Source: CAD feature listing. Evaluate the final solid. Frame: model axes, mm. Face numbers are marked on the shaded views. A direction names the side the tool comes from. Give positions to 0.01 mm unless a question says otherwise; leave off trailing zeros. Order: outer loops, then holes, each group sorted by start corner. A loop starts at its lowest first (then second) coordinate and runs counter-clockwise, first axis right, second up.
```python
from build123d import *

# Parameters (mm, degrees)
SKETCH_1_W          = 640
SKETCH_1_H          = 75
EXTRUDE_1_DEPTH     = 3
SKETCH_2_W          = 640
SKETCH_2_H          = 3
EXTRUDE_2_DEPTH     = 17
FILLET_1_R          = 5
SKETCH_5_R          = 2.5
CUT_EXTRUDE_3_DEPTH = 645.347732207
SKETCH_3_R          = 3.25
CUT_EXTRUDE_1_DEPTH = 645.603754255
SKETCH_4_W          = 20.5
SKETCH_4_H          = 72
CUT_EXTRUDE_2_DEPTH = 645.603754255
FILLET_3_R          = 2


with BuildPart() as part:
    # 스케치1 → 보스-돌출1 (new body)
    with BuildSketch(Plane.XY):
        with Locations((320, 37.5)):
            Rectangle(SKETCH_1_W, SKETCH_1_H)
    extrude(amount=EXTRUDE_1_DEPTH)

    # 스케치2 → 보스-돌출2 (add)
    with BuildSketch(Plane.XY.offset(3)):
        with Locations((320, 73.5)):
            Rectangle(SKETCH_2_W, SKETCH_2_H)
    extrude(amount=EXTRUDE_2_DEPTH)

    # 필렛1
    fillet_1_edges = [part.edges().sort_by_distance(p)[0] for p in [
        (320, 75, 0),
    ]]
    fillet(fillet_1_edges, radius=FILLET_1_R)

    # 스케치5 → 컷-돌출3 (cut, through all)
    with BuildSketch(Plane.XZ.offset(-72)):
        with Locations(Location((60, 11.5, 0), (0, 0, 270))):
            Circle(SKETCH_5_R)
        with Locations(Location((580, 11.5, 0), (0, 0, 270))):
            Circle(SKETCH_5_R)
    extrude(amount=-CUT_EXTRUDE_3_DEPTH, mode=Mode.SUBTRACT)

    # 스케치3 → 컷-돌출1 (cut, through all)
    with BuildSketch(Plane.XY.offset(3)):
        with Locations((80, 55)):
            Circle(SKETCH_3_R)
        with Locations((80, 20)):
            Circle(SKETCH_3_R)
        with Locations((320, 55)):
            Circle(SKETCH_3_R)
        with Locations((320, 20)):
            Circle(SKETCH_3_R)
        with Locations((560, 55)):
            Circle(SKETCH_3_R)
        with Locations((560, 20)):
            Circle(SKETCH_3_R)
    extrude(amount=-CUT_EXTRUDE_1_DEPTH, mode=Mode.SUBTRACT)

    # 스케치4 → 컷-돌출2 (cut, through all)
    with BuildSketch(Plane.XY.offset(3)):
        with Locations((10.25, 36)):
            Rectangle(SKETCH_4_W, SKETCH_4_H)
        with Locations((629.75, 36)):
            Rectangle(SKETCH_4_W, SKETCH_4_H)
    extrude(amount=-CUT_EXTRUDE_2_DEPTH, mode=Mode.SUBTRACT)

    # 필렛3
    fillet_3_edges = [part.edges().sort_by_distance(p)[0] for p in [
        (320, 72, 3),
    ]]
    fillet(fillet_3_edges, radius=FILLET_3_R)


solid = part.part
```
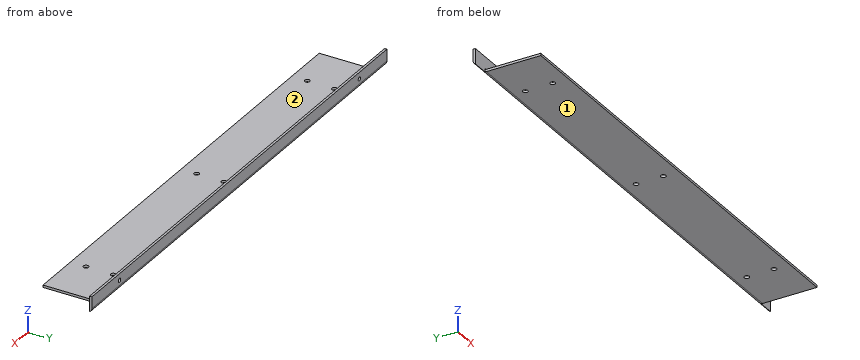
1) Reachability of the marked faces 1 and 2 from +Z, -Z, +X, -X, +Y, -Y: full face, straight path, thin tool, end or side. Return the list, or none.
Report:
face 1: -Z, +X, -X, +Y, -Y
face 2: +Z, +X, -X, -Y
2) Pin query (flat end, axial travel): pin 1 (5 mm diameter, centred on x = 320, y = 20, fed in from -Z); pin 2 (2.5 mm diameter, centred on y = 20.5, z = 1.5, fed in from -X); pin 3 (7.5 mm diameter, centred on x = 80, y = 55, fed in from +Z); pin 4 (4 mm diameter, centred on y = 47, z = 3, fed in from +X). Return the tip coordinate at first contact, or that it passes through.
Report:
pin 1: passes through
pin 2: stops at x = 20.5
pin 3: stops at z = 3
pin 4: stops at x = 619.5
3) Section query A-A, the plane x = 521.5. Return the cut outline in (y, z), and give its area (3 significant figures).
Report:
outline: (0, 0) - (70, 0) arc R5 ccw to (75, 5) - (75, 20) - (72, 20) - (72, 5) arc R2 cw to (70, 3) - (0, 3) - close
area: 271 mm2
4) Material intervals for L1, parallel to X at y = 74, z = 11.5; L2, parallel to X at y = 54, z = 1; L3, parallel to Z at x = 497.5, y = 55.5, sorted ascending.
Report:
L1: x = 0 to 57.5, 62.5 to 577.5, 582.5 to 640
L2: x = 20.5 to 76.91, 83.09 to 316.91, 323.09 to 556.91, 563.09 to 619.5
L3: z = 0 to 3
5) Section query B-B, the plane y = 34. Return the cut outline in (x, z).
Report:
outline: (20.5, 0) - (619.5, 0) - (619.5, 3) - (20.5, 3) - close
